from build123d import *

# Parameters (mm, degrees)
SKETCH1_R           = 14.2875
BOSS_EXTRUDE1_DEPTH = 38.1
SKETCH2_W           = 76.2
SKETCH2_H           = 38.1
SKETCH2_R           = 14.2875
BOSS_EXTRUDE2_DEPTH = 38.1
CUT_EXTRUDE1_DEPTH  = 38.1
FILLET1_R           = 12.7


with BuildPart() as part:
    # Sketch1 → Boss-Extrude1 (new body)
    with BuildSketch(Plane(origin=(0, 0, 0), x_dir=(0, 0, -1), z_dir=(1, 0, 0))):
        with BuildLine():
            Line((29.337186502, -19.05), (-175.255687154, -19.05))
            Line((-175.255687154, -19.05), (-175.255687154, 19.05))
            Line((-175.255687154, 19.05), (29.337186502, 19.05))
            Line((29.337186502, 19.05), (29.337186502, 4))
            Line((29.337186502, 4), (13.442493258, 4))
            ThreePointArc((13.442493258, 4), (0, 14.025), (-13.442493258, 4))
            Line((-13.442493258, 4), (-18.025, 4))
            Line((-18.025, 4), (-18.025, -4))
            Line((-18.025, -4), (-13.442493258, -4))
            ThreePointArc((-13.442493258, -4), (0, -14.025), (13.442493258, -4))
            Line((13.442493258, -4), (29.337186502, -4))
            Line((29.337186502, -4), (29.337186502, -19.05))
        make_face()
        with Locations(Location((-152.4, 0, 0), (0, 0, 180))):
            Circle(SKETCH1_R, mode=Mode.SUBTRACT)
    extrude(amount=BOSS_EXTRUDE1_DEPTH)

    # Sketch2 → Boss-Extrude2 (add)
    with BuildSketch(Plane(origin=(38.1, 0, 0), x_dir=(0, 0, -1), z_dir=(1, 0, 0))):
        with Locations((-137.155687154, 0)):
            Rectangle(SKETCH2_W, SKETCH2_H)
        with Locations(Location((-152.4, 0, 0), (0, 0, 180))):
            Circle(SKETCH2_R, mode=Mode.SUBTRACT)
    extrude(amount=BOSS_EXTRUDE2_DEPTH)

    # Sketch3 → Cut-Extrude1 (cut)
    with BuildSketch(Plane(origin=(0, 19.05, 0), x_dir=(1, 0, 0), z_dir=(0, 1, 0))):
        Polygon((38.1, -99.055687154), (76.2, -132.562404594), (94.277321555, -84.449227978), align=None)
    extrude(amount=-CUT_EXTRUDE1_DEPTH, mode=Mode.SUBTRACT)

    # Fillet1
    fillet1_edges = [part.edges().sort_by_distance(p)[0] for p in [
        (38.1, 0, 99.055687154),
    ]]
    fillet(fillet1_edges, radius=FILLET1_R)


solid = part.part
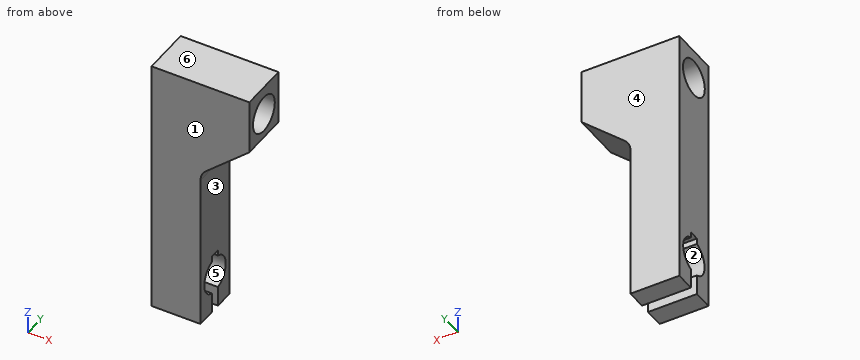
Model file for the job. Use its own axes, mm. Face numbers are marked on the shaded views. A direction names the side the tool comes from. Give positions to 0.01 mm unless a question says otherwise; leave off trailing zeros. Loops run counter-clockwise (first coordinate to the right, second up) from the corner with the lowest first, then second, coordinate; pieces in that order, holes last.
1) Saw through at C-C (y = 0). Write the cut outline in (x, z) (1 decimal), plus the area to 3 significant figures.
2) Saw through at B-B (z = 4). Write the cut outline in (x, y).
3) Saw through at D-D (z = 152.4). Write the cut outline in (x, y), plus the area to 3 significant figures.
4) Pull direction Z, two halves, no side cores. Call the marked faces 4, 5 and 6: +Z half, -Z half, draft (parallel to the pull), parting line (faces both ways), or undercut.
5) Flat gauge pins, fed straight in: pin 1 Ø8 at (y, z) = (6.5, 110.5) entering from +X; pin 2 Ø4 at (x, y) = (31, 1.5) entering from -Z (3 decimals); pin 3 Ø2 at (y, z) = (0.5, 39.5) entering from +X. Where does each tip first touch, or does it go through?
6) Wall check: line 1 (Y direction, x = 60, z = 152.4); line 2 (Z direction, x = 25, y = 6.5); line 3 (Y direction, x = 29.5, z = 157). Give the ranges that are in metal, low to high.
7) Tool access for the marked faces 1, 2 and 3: list every direction of +Z, -Z, +X, -X, +Y, -Y with a clear straight run to the whole face (end or side of a thin tool).
Answer block:
1. outline: (0, 18) - (38.1, 18) - (38.1, 93.3) arc R12.7 cw to (42.4, 102.8) - (76.2, 132.6) - (76.2, 138.1) - (0, 138.1) - close; (0, 166.7) - (76.2, 166.7) - (76.2, 175.3) - (0, 175.3) - close
1. area: 6,080 mm2
2. outline: (0, -19.05) - (38.1, -19.05) - (38.1, -13.44) - (0, -13.44) - close; (0, 13.44) - (38.1, 13.44) - (38.1, 19.05) - (0, 19.05) - close
3. outline: (0, -19.05) - (76.2, -19.05) - (76.2, -14.29) - (0, -14.29) - close; (0, 14.29) - (76.2, 14.29) - (76.2, 19.05) - (0, 19.05) - close
3. area: 726 mm2
4. face 4: draft
4. face 5: undercut
4. face 6: +Z half
5. pin 1: stops at x = 55.66
5. pin 2: stops at z = 18.025
5. pin 3: stops at x = 38.1
6. line 1: y = -19.05 to -14.29, 14.29 to 19.05
6. line 2: z = -29.34 to -12.43, 12.43 to 139.68, 165.12 to 175.26
6. line 3: y = -19.05 to -13.53, 13.53 to 19.05
7. face 1: +Z, -Z, +X, -X, -Y
7. face 2: +X, -X
7. face 3: -Z, +X, +Y, -Y
